from build123d import *

# Parameters (mm, degrees)
CROQUIS1_R              = 24.4
SALIENTE_EXTRUIR1_DEPTH = 70
SALIENTE_EXTRUIR2_START = -4
CROQUIS2_R              = 27.5
CROQUIS2_R_2            = 24.4
SALIENTE_EXTRUIR2_DEPTH = 4
SALIENTE_EXTRUIR3_START = 10
CROQUIS3_R              = 27.5
CROQUIS3_R_2            = 25.4
SALIENTE_EXTRUIR3_DEPTH = 10


with BuildPart() as part:
    # Croquis1 → Saliente-Extruir1 (new body)
    with BuildSketch(Plane(origin=(0, 0, 0), x_dir=(0, 0, -1), z_dir=(1, 0, 0))):
        Circle(CROQUIS1_R)
        Polygon((7.332348419, 0), (3.666174209, 6.35), (-3.666174209, 6.35), (-7.332348419, 0), (-3.666174209, -6.35), (3.666174209, -6.35), align=None, mode=Mode.SUBTRACT)
    extrude(amount=SALIENTE_EXTRUIR1_DEPTH)

    # Croquis2 → Saliente-Extruir2 (add)
    with BuildSketch(Plane(origin=(70, 0, 0), x_dir=(0, 0, -1), z_dir=(1, 0, 0)).offset(SALIENTE_EXTRUIR2_START)):
        Circle(CROQUIS2_R)
        Circle(CROQUIS2_R_2, mode=Mode.SUBTRACT)
    extrude(amount=SALIENTE_EXTRUIR2_DEPTH)

    # Croquis3 → Saliente-Extruir3 (add)
    with BuildSketch(Plane.ZY.offset(-66).offset(SALIENTE_EXTRUIR3_START)):
        with Locations(Location((0, 0, 0), (0, 0, 180))):
            Circle(CROQUIS3_R)
        Circle(CROQUIS3_R_2, mode=Mode.SUBTRACT)
    extrude(amount=-SALIENTE_EXTRUIR3_DEPTH)


solid = part.part
Could you check a few things on this model? Use its own coordinates, in mm. A direction names the side the tool comes from. Give positions to 0.01 mm unless a question says otherwise; leave off trailing zeros. Order: outer loops, then holes, each group sorted by start corner. A loop starts at its lowest first (then second) coordinate and runs counter-clockwise, first axis right, second up. Notation, with made-up numbers: (-31.5, 22) -> (-19.5, 22) arc R22 ccw to (-19.5, 49) -> close; hole circle Ø5 at (-40, 83). An arc over 180 degrees is marked (long way). Return JSON: item names as keys, results as strings.
1. Imagine slicing it at D-D on y = -11. List the corners of the cut face in (x, z) for me.
Answer list:
{"outline": "(0, -21.78) -> (66, -21.78) -> (66, -22.89) -> (56, -22.89) -> (56, -25.2) -> (70, -25.2) -> (70, 25.2) -> (56, 25.2) -> (56, 22.89) -> (66, 22.89) -> (66, 21.78) -> (0, 21.78) -> close"}
2. On a 3-axis mill with a long thin cutter (end or side, diameter ignored), from which of +Z, -Z, +X, -X, +Y, -Y can I reach the whole of each face in a straight line? I mean faces 1 (the flat face through (34.51, -3.219, -5.474)), 2 (the cylindrical face through (32.538, 1.073, 24.376)), 3 (the flat face through (0, -5, -5)). Say none if no direction works.
Answer list:
{"face 1": "+X, -X", "face 2": "-X", "face 3": "+Z, -Z, -X, +Y, -Y"}
3. For pin 1 Ø8 at (x, z) = (19.5, -0.5) entering from -Y; pin 2 Ø2 at (x, z) = (19, 1) entering from +Y; pin 3 Ø6 at (x, z) = (41.5, 16.5) entering from -Y, each with a flat end and sliding along its axis, tell me the tip position at first contact or that it passes through.
Answer list:
{"pin 1": "stops at y = -24.4", "pin 2": "stops at y = 24.4", "pin 3": "stops at y = -20.33"}
4. Imagine slicing it at C-C on x = 6. List the corners of the cut face in (y, z) for me.
Answer list:
{"outline": "circle Ø48.8 at (0, 0); hole (-6.35, -3.67) -> (0, -7.33) -> (6.35, -3.67) -> (6.35, 3.67) -> (0, 7.33) -> (-6.35, 3.67) -> close"}
5. I need wall thicknesses on line 1 (Y direction, x = 62.5, z = 0); line 2 (Z direction, x = 64.5, y = 15.5); line 3 (Y direction, x = 62, z = -5). Which ranges of each line are inside material? Lowest first, please. Write a range as from..to.
Answer list:
{"line 1": "y = -27.5..-25.4, -24.4..-6.35, 6.35..24.4, 25.4..27.5", "line 2": "z = -22.72..-20.12, -18.84..18.84, 20.12..22.72", "line 3": "y = -27.04..-24.9, -23.88..-4.04, 4.04..23.88, 24.9..27.04"}
6. Imagine slicing it at B-B on x = 63. List the corners of the cut face in (y, z) for me.
Answer list:
{"outline": "circle Ø55 at (0, 0); circle Ø48.8 at (0, 0); hole circle Ø50.8 at (0, 0); hole (-6.35, -3.67) -> (0, -7.33) -> (6.35, -3.67) -> (6.35, 3.67) -> (0, 7.33) -> (-6.35, 3.67) -> close"}
7. Thinking about a two-plate mould opening in Z: for faces 4 (the cylindrical face through (62.902, 24.397, -12.69)), 5 (the flat face through (70, 6.5, 0.4)), 6 (the flat face through (34.51, 3.131, -5.525)), which applies, pulls with the +Z half, pulls with the -Z half, needs draft (parallel to the pull), parting line crosses it, or undercut?
Answer list:
{"face 4": "parting line crosses it", "face 5": "needs draft", "face 6": "undercut"}
8. Imagine slicing it at A-A on z = 0. List the corners of the cut face in (x, y) for me, then the cut area to 3 significant figures.
Answer list:
{"outline": "(0, -24.4) -> (66, -24.4) -> (66, -25.4) -> (56, -25.4) -> (56, -27.5) -> (70, -27.5) -> (70, -6.35) -> (0, -6.35) -> close; (0, 6.35) -> (70, 6.35) -> (70, 27.5) -> (56, 27.5) -> (56, 25.4) -> (66, 25.4) -> (66, 24.4) -> (0, 24.4) -> close", "area": "2,590 mm2"}
